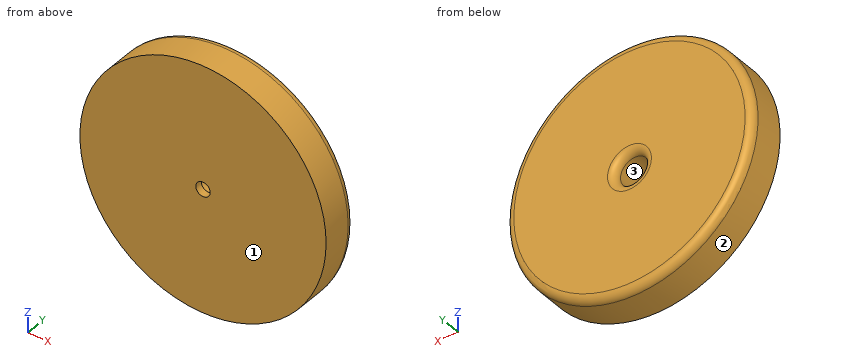
from build123d import *

# Parameters (mm, degrees)
SKETCH1_R           = 33.072163115
BOSS_EXTRUDE1_DEPTH = 10
SKETCH2_R           = 3.89
CUT_EXTRUDE1_DEPTH  = 8
SKETCH3_R           = 1.935
CUT_EXTRUDE2_DEPTH  = 8
FILLET1_R           = 2
FILLET2_R           = 2


with BuildPart() as part:
    # Sketch1 → Boss-Extrude1 (new body)
    with BuildSketch(Plane(origin=(0, 0, 0), x_dir=(1, 0, 0), z_dir=(0, 1, 0))):
        Circle(SKETCH1_R)
    extrude(amount=BOSS_EXTRUDE1_DEPTH)

    # Sketch2 → Cut-Extrude1 (cut)
    with BuildSketch(Plane(origin=(0, 10, 0), x_dir=(1, 0, 0), z_dir=(0, 1, 0))):
        Circle(SKETCH2_R)
    extrude(amount=-CUT_EXTRUDE1_DEPTH, mode=Mode.SUBTRACT)

    # Sketch3 → Cut-Extrude2 (cut)
    with BuildSketch(Plane(origin=(0, 2, 0), x_dir=(1, 0, 0), z_dir=(0, 1, 0))):
        Circle(SKETCH3_R)
    extrude(amount=-CUT_EXTRUDE2_DEPTH, mode=Mode.SUBTRACT)

    # Fillet1
    fillet1_edges = [part.edges().sort_by_distance(p)[0] for p in [
        (-33.072163115, 10, 0),
    ]]
    fillet(fillet1_edges, radius=FILLET1_R)

    # Fillet2
    fillet2_edges = [part.edges().sort_by_distance(p)[0] for p in [
        (-3.89, 10, 0),
    ]]
    fillet(fillet2_edges, radius=FILLET2_R)


solid = part.part
The model under review builds one solid part; all positions refer to its coordinate system, in mm. Face numbers are marked on the shaded views. Give positions to 0.01 mm unless a question says otherwise; leave off trailing zeros. Loops run counter-clockwise (first coordinate to the right, second up) from the corner with the lowest first, then second, coordinate; pieces in that order, holes last. Notation, with made-up numbers: (-2, 61.5) -> (31, 61.5) arc R30 ccw to (31, 97.5) -> close; hole circle Ø2 at (18, 40.5). An arc over 180 degrees is marked (long way). Answer as a JSON object with one key per item and string values. Group by question number.
Q1. Insertion check: pin 1 (3 mm diameter, centred on x = -12, z = -2, fed in from -Y); pin 2 (2.5 mm diameter, centred on x = 2, z = 1.5, fed in from +Y); pin 3 (3 mm diameter, centred on x = -12.5, y = 7.5, fed in from -Z); pin 4 (5 mm diameter, centred on x = -15, y = 9, fed in from -Z). Each pin has a flat end and moves straight along its axis. Give the tip position at first contact, or say it passes through.
Q2. Take a section at A-A (x = 0). Write out the cut boundary in (y, z) (3 decimals).
Q3. Take a section at B-B (z = 0). Write out the cut boundary in (x, y) (3 decimals).
Q4. Take a section at C-C (y = 6.75). Write out the cut boundary in (x, z), plus the area to 3 significant figures.
Q5. Wall thickness on line 1 along Z through (x, y) = (0, 1.1) (3 decimals); line 2 along X through (y, z) = (6.25, 0); line 3 along Z through (x, y) = (-2, 7.25): over which ranges is each line inside the solid? List them lowest first.
Q6. Draft analysis for pull direction X (two halves, no side actions). For the marked faces 1, 2 and 3, state which applies: pulls with the +X half, pulls with the -X half, needs draft (parallel to the pull), parting line crosses it, or undercut.
Answer below:
{
 "1": {"pin 1": "stops at y = 0", "pin 2": "stops at y = 2", "pin 3": "stops at z = -31.19", "pin 4": "stops at z = -30.55"},
 "2": {"outline": "(0, -33.072) -> (8, -33.072) arc R2 ccw to (10, -31.072) -> (10, -5.89) arc R2 ccw to (8, -3.89) -> (2, -3.89) -> (2, -1.935) -> (0, -1.935) -> close; (0, 1.935) -> (2, 1.935) -> (2, 3.89) -> (8, 3.89) arc R2 ccw to (10, 5.89) -> (10, 31.072) arc R2 ccw to (8, 33.072) -> (0, 33.072) -> close"},
 "3": {"outline": "(-33.072, 0) -> (-1.935, 0) -> (-1.935, 2) -> (-3.89, 2) -> (-3.89, 8) arc R2 ccw to (-5.89, 10) -> (-31.072, 10) arc R2 ccw to (-33.072, 8) -> close; (1.935, 0) -> (33.072, 0) -> (33.072, 8) arc R2 ccw to (31.072, 10) -> (5.89, 10) arc R2 ccw to (3.89, 8) -> (3.89, 2) -> (1.935, 2) -> close"},
 "4": {"outline": "circle Ø66.14 at (0, 0); hole circle Ø7.78 at (0, 0)", "area": "3,390 mm2"},
 "5": {"line 1": "z = -33.072 to -1.935, 1.935 to 33.072", "line 2": "x = -33.07 to -3.89, 3.89 to 33.07", "line 3": "z = -33.01 to -3.34, 3.34 to 33.01"},
 "6": {"face 1": "needs draft", "face 2": "parting line crosses it", "face 3": "undercut"}
}
